```python
from build123d import *

# Parameters (mm, degrees)
BOSS_EXTRUDE1_DEPTH        = 2
M2_CLEARANCE_HOLE1_D       = 2.459
M3_CLEARANCE_HOLE1_D       = 3.242
SKETCHED_START             = 39.700827994
SKETCHED_BEND1_OUTLINE_W   = 2
SKETCHED_BEND1_OUTLINE_H   = 25.75
SKETCHED_BEND1_DEPTH       = 17.149172006
SKETCHED_START_2           = 36.111787994
SKETCHED_BEND1_2_DEPTH     = 4
SKETCHED_START_3           = -5.75
SKETCHED_BEND1_3_DEPTH     = 25.75
SKETCHED_START_4           = -18.6
SKETCHED_BEND2_OUTLINE_W   = 2
SKETCHED_BEND2_OUTLINE_H   = 40
SKETCHED_BEND2_DEPTH       = 19.122747994
SKETCHED_START_5           = 0.752486697
SKETCHED_BEND2_2_OUTLINE_R = 1.621
SKETCHED_BEND2_2_DEPTH     = 1.359301297
SKETCHED_START_6           = 0.111787994
SKETCHED_BEND2_3_OUTLINE_R = 1.621
SKETCHED_BEND2_3_DEPTH     = 4
SKETCHED_START_7           = -20
SKETCHED_BEND2_4_DEPTH     = 40


with BuildPart() as part:
    # Sketch7 → Boss-Extrude1 (new body)
    with BuildSketch(Plane.XZ):
        with BuildLine():
            Line((35.65, -5.75), (52.85, -5.75))
            ThreePointArc((52.85, -5.75), (55.678427125, -4.578427125), (56.85, -1.75))
            Line((56.85, -1.75), (56.85, 16))
            ThreePointArc((56.85, 16), (55.678427125, 18.828427125), (52.85, 20))
            Line((52.85, 20), (-14.6, 20))
            ThreePointArc((-14.6, 20), (-17.428427125, 18.828427125), (-18.6, 16))
            Line((-18.6, 16), (-18.6, -16))
            ThreePointArc((-18.6, -16), (-17.428427125, -18.828427125), (-14.6, -20))
            Line((-14.6, -20), (33.65, -20))
            ThreePointArc((33.65, -20), (35.064213562, -19.414213562), (35.65, -18))
            Line((35.65, -18), (35.65, -5.75))
        make_face()
    extrude(amount=-BOSS_EXTRUDE1_DEPTH)

    # M2 Clearance Hole1 (through all)
    with Locations(Plane(origin=(0, 0, 0), x_dir=(-1, 0, 0), z_dir=(0, -1, 0))):
        with Locations((-33.1, 16), (-33.1, -2.75)):
            Hole(M2_CLEARANCE_HOLE1_D / 2)

    # M3 Clearance Hole1 (through all)
    with Locations(Plane(origin=(0, 2, 0), x_dir=(1, 0, 0), z_dir=(0, 1, 0))):
        with Locations((-11.65, -15), (-11.65, 15)):
            Hole(M3_CLEARANCE_HOLE1_D / 2)

    # Sketched Bend1: read off the stored shape, not the designer's step
    # Sketched Bend1 outline → Sketched Bend1 (cut)
    with BuildSketch(Plane.YZ.offset(SKETCHED_START)):
        with Locations((1, 7.125)):
            Rectangle(SKETCHED_BEND1_OUTLINE_W, SKETCHED_BEND1_OUTLINE_H)
    extrude(amount=SKETCHED_BEND1_DEPTH, mode=Mode.SUBTRACT)

    # Sketched Bend1 2 outline → Sketched Bend1 2 (add)
    with BuildSketch(Plane.YZ.offset(SKETCHED_START_2)):
        with BuildLine():
            Line((0, 20), (-14.025823026, 20))
            ThreePointArc((-14.025823026, 20), (-16.854250151, 18.828427124), (-18.025823026, 16))
            Line((-18.025823026, 16), (-18.025823026, -1.75))
            ThreePointArc((-18.025823026, -1.75), (-16.854250151, -4.578427124), (-14.025823026, -5.75))
            Line((-14.025823026, -5.75), (0, -5.75))
            Line((0, -5.75), (0, 20))
        make_face()
    extrude(amount=SKETCHED_BEND1_2_DEPTH)

    # Sketched Bend1 3 outline → Sketched Bend1 3 (cut)
    with BuildSketch(Plane.XY.offset(SKETCHED_START_3)):
        with BuildLine():
            ThreePointArc((36.111787994, 2), (38.940215119, 0.828427125), (40.111787994, -2))
            Line((40.111787994, -2), (40.111787994, 0))
            Line((40.111787994, 0), (39.700827994, 0))
            Line((39.700827994, 0), (39.700827994, 2))
            Line((39.700827994, 2), (36.111787994, 2))
        make_face()
        with BuildLine():
            Line((38.111787994, -18.025823026), (38.111787994, -2))
            ThreePointArc((38.111787994, -2), (37.526001556, -0.585786438), (36.111787994, 0))
            Line((36.111787994, 0), (36.111787994, -18.025823026))
            Line((36.111787994, -18.025823026), (38.111787994, -18.025823026))
        make_face()
    extrude(amount=SKETCHED_BEND1_3_DEPTH, mode=Mode.SUBTRACT)

    # Sketched Bend2: read off the stored shape, not the designer's step
    # Sketched Bend2 outline → Sketched Bend2 (cut)
    with BuildSketch(Plane.YZ.offset(SKETCHED_START_4)):
        with Locations((1, 0)):
            Rectangle(SKETCHED_BEND2_OUTLINE_W, SKETCHED_BEND2_OUTLINE_H)
    extrude(amount=SKETCHED_BEND2_DEPTH, mode=Mode.SUBTRACT)

    # Sketched Bend2 2 outline → Sketched Bend2 2 (add)
    with BuildSketch(Plane.YZ.offset(SKETCHED_START_5)):
        with BuildLine():
            Line((0, 20), (-15.999399014, 20))
            ThreePointArc((-15.999399014, 20), (-18.827826139, 18.828427125), (-19.999399014, 16))
            Line((-19.999399014, 16), (-19.999399014, -16))
            ThreePointArc((-19.999399014, -16), (-18.827826139, -18.828427124), (-15.999399014, -20))
            Line((-15.999399014, -20), (0, -20))
            Line((0, -20), (0, 20))
        make_face()
        with Locations((-13.049399014, -15)):
            Circle(SKETCHED_BEND2_2_OUTLINE_R, mode=Mode.SUBTRACT)
        with Locations((-13.049399014, 15)):
            Circle(SKETCHED_BEND2_2_OUTLINE_R, mode=Mode.SUBTRACT)
    extrude(amount=SKETCHED_BEND2_2_DEPTH)

    # Sketched Bend2 3 outline → Sketched Bend2 3 (add)
    with BuildSketch(Plane.YZ.offset(SKETCHED_START_6)):
        with BuildLine():
            Line((0, 20), (-15.999399014, 20))
            ThreePointArc((-15.999399014, 20), (-18.827826139, 18.828427125), (-19.999399014, 16))
            Line((-19.999399014, 16), (-19.999399014, -16))
            ThreePointArc((-19.999399014, -16), (-18.827826139, -18.828427124), (-15.999399014, -20))
            Line((-15.999399014, -20), (0, -20))
            Line((0, -20), (0, 20))
        make_face()
        with Locations((-13.049399014, -15)):
            Circle(SKETCHED_BEND2_3_OUTLINE_R, mode=Mode.SUBTRACT)
        with Locations((-13.049399014, 15)):
            Circle(SKETCHED_BEND2_3_OUTLINE_R, mode=Mode.SUBTRACT)
    extrude(amount=SKETCHED_BEND2_3_DEPTH)

    # Sketched Bend2 4 outline → Sketched Bend2 4 (cut)
    with BuildSketch(Plane.XY.offset(SKETCHED_START_7)):
        with BuildLine():
            Line((0.111787994, 0), (0.111787994, -2))
            ThreePointArc((0.111787994, -2), (1.283360869, 0.828427125), (4.111787994, 2))
            Line((4.111787994, 2), (0.522747994, 2))
            Line((0.522747994, 2), (0.522747994, 0))
            Line((0.522747994, 0), (0.111787994, 0))
        make_face()
        with BuildLine():
            ThreePointArc((4.111787994, 0), (2.697574432, -0.585786438), (2.111787994, -2))
            Line((2.111787994, -2), (2.111787994, -19.999399014))
            Line((2.111787994, -19.999399014), (4.111787994, -19.999399014))
            Line((4.111787994, -19.999399014), (4.111787994, 0))
        make_face()
    extrude(amount=SKETCHED_BEND2_4_DEPTH, mode=Mode.SUBTRACT)


solid = part.part
```
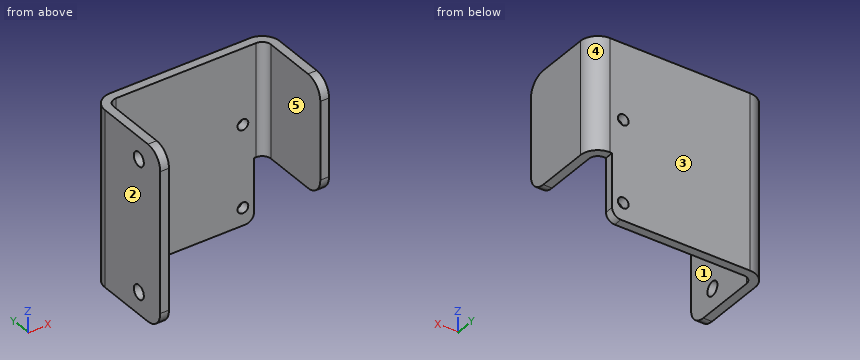
The model under review builds one solid part; all positions refer to its coordinate system, in mm. Face numbers are marked on the shaded views. A direction names the side the tool comes from. Give positions to 0.01 mm unless a question says otherwise; leave off trailing zeros. Write each loop counter-clockwise with the first axis right and the second up, starting at its lowest first coordinate (ties: lowest second). Pieces come first, ordered by that corner, then holes. Notation, with made-up numbers: M 23,33.5 L 53,33.5 A5 ccw 53,40.5 Z; hole C 19.5,48 d4. An arc over 180 degrees is marked long. Write item = value, one per line. Start each with the question number.
Q1. For line 1 (Z direction, x = 33.1, y = 1.15); line 2 (X direction, y = -16.5, z = 11.5); line 3 (Y direction, x = 23.5, z = 5.5), list the stretches that pass through material, from the lowest coordinate up.
Q2. We need section C-C (x = 33.1). State the section outline as (y, z) points.
Q3. We need section D-D (z = 0.5). State the section outline as (x, y) points.
Q4. We need section B-B (z = 15). State the section outline as (x, y) points.
Q5. We need section A-A (y = -9.75). State the section outline as (x, z) points, plus the area to 4 significant figures.
Q6. Machinability: for the marked faces 1 and 2, which of the approach directions +Z, -Z, +X, -X, +Y, -Y give a long, thin tool a straight path to every point of the face, cutting with its end or side? Answer none if there is none.
Q7. Mouldability with a two-part tool opening along X and no side actions: class the marked faces 3, 4 and 5 as released by +X, released by -X, zero draft, split by the parting line, or undercut.
Q8. Clearance check with flat-ended pins moving along their axes: pin 1 (0.6 mm diameter, centred on y = 1, z = -13.5, fed in from +X); pin 2 (1.3 mm diameter, centred on x = 38, y = -3, fed in from -Z); pin 3 (5 mm diameter, centred on y = -13.05, z = -15, fed in from +X). State where each tip first meets the part, or that it passes through.
Result set:
q1.line_1 = -20 to -17.23, -14.77 to 1.52, 3.98 to 20
q1.line_2 = 0.11 to 2.11, 38.11 to 40.11
q1.line_3 = 0 to 2
q2.outline = M 0,-20 L 2,-20 L 2,-17.23 L 0,-17.23 Z; M 0,-14.77 L 2,-14.77 L 2,1.52 L 0,1.52 Z; M 0,3.98 L 2,3.98 L 2,20 L 0,20 Z
q3.outline = M 0.11,-20 L 2.11,-20 L 2.11,-2 A2 cw 4.11,0 L 36.11,0 A2 cw 38.11,-2 L 38.11,-18.03 L 40.11,-18.03 L 40.11,-2 A4 ccw 36.11,2 L 4.11,2 A4 ccw 0.11,-2 Z
q4.outline = M 0.11,-20 L 2.11,-20 L 2.11,-14.67 L 0.11,-14.67 Z; M 0.11,-11.43 L 2.11,-11.43 L 2.11,-2 A2 cw 4.11,0 L 36.11,0 A2 cw 38.11,-2 L 38.11,-18.03 L 40.11,-18.03 L 40.11,-2 A4 ccw 36.11,2 L 4.11,2 A4 ccw 0.11,-2 Z
q5.outline = M 0.11,-20 L 2.11,-20 L 2.11,20 L 0.11,20 Z; M 38.11,-5.75 L 40.11,-5.75 L 40.11,20 L 38.11,20 Z
q5.area = 131.5 mm2
q6.face_1 = +Z, -Z, -Y
q6.face_2 = +Z, -Z, -X, +Y, -Y
q7.face_3 = zero draft
q7.face_4 = released by +X
q7.face_5 = undercut
q8.pin_1 = 35.65
q8.pin_2 = -5.75
q8.pin_3 = 2.11
